```python
from build123d import *

# Parameters (mm, degrees)
SKETCH_1_W             = 10
SKETCH_1_H             = 40
SKETCH_1_R             = 1.5
EXTRUDE_1_DEPTH        = 3
SKETCH_2_W             = 1.55
SKETCH_2_H             = 40
EXTRUDE_2_DEPTH        = 3
CUT_EXTRUDE_1_DEPTH    = 3
PATTERN_LINEAR_1_COUNT = 40
PATTERN_LINEAR_1_PITCH = 1
CUT_EXTRUDE_2_DEPTH    = 10
FILLET_1_R             = 1
CUT_EXTRUDE_3_DEPTH    = 10
FILLET_2_R             = 1


with BuildPart() as part:
    # 草图1 → 凸台-拉伸1 (new body)
    with BuildSketch(Plane.XY):
        Rectangle(SKETCH_1_W, SKETCH_1_H)
        Circle(SKETCH_1_R, mode=Mode.SUBTRACT)
    extrude(amount=EXTRUDE_1_DEPTH)

    # 草图2 → 凸台-拉伸2 (add)
    with BuildSketch(Plane.XY.offset(3)):
        with Locations((-5.775, 0)):
            Rectangle(SKETCH_2_W, SKETCH_2_H)
    extrude(amount=-EXTRUDE_2_DEPTH)

    # 草图3 → 切除-拉伸1 (cut)
    with BuildSketch(Plane.XY.offset(3)):
        Polygon((-6.55, 19.8), (-6.05, 19.566846171), (-6.55, 19.333692342), align=None)
    cut_extrude_1 = extrude(amount=-CUT_EXTRUDE_1_DEPTH, mode=Mode.SUBTRACT)

    # 阵列(线性)1: 切除-拉伸1 ×40
    with Locations(*[(0, -i * PATTERN_LINEAR_1_PITCH, 0) for i in range(1, PATTERN_LINEAR_1_COUNT)]):
        add(cut_extrude_1, mode=Mode.SUBTRACT)

    # 草图5 → 切除-拉伸2 (cut)
    with BuildSketch(Plane.XY.offset(3)):
        Polygon((-0.5, 20), (-0.5, 8.485281374), (-5, 3), (-5.480467746, 6.547419937), (-7.040068743, 6.547419937), (-7.040068743, 9.445607815), (-8.18437591, 20), align=None)
    extrude(amount=-CUT_EXTRUDE_2_DEPTH, mode=Mode.SUBTRACT)

    # 圆角1
    fillet_1_edges = [part.edges().sort_by_distance(p)[0] for p in [
        (-0.5, 8.485281374, 1.5),
        (-5, 3, 1.5),
    ]]
    fillet(fillet_1_edges, radius=FILLET_1_R)

    # 草图7 → 切除-拉伸3 (cut)
    with BuildSketch(Plane(origin=(0, 0, 0), x_dir=(-1, 0, 0), z_dir=(0, 0, -1))):
        with BuildLine():
            Line((6.55, -20), (-5.418170251, -22.566873238))
            Line((-5.418170251, -22.566873238), (-10.062870934, -14.075772272))
            Line((-10.062870934, -14.075772272), (-5, -10.23011241))
            add(Edge.make_bspline(
                [(-5, -10.23011241), (-3.025837533, -19.554793567), (6.55, -20)],
                knots=[0, 0, 0, 1, 1, 1], degree=2))
        make_face()
    extrude(amount=-CUT_EXTRUDE_3_DEPTH, mode=Mode.SUBTRACT)

    # 圆角2
    fillet_2_edges = [part.edges().sort_by_distance(p)[0] for p in [
        (-0.5, 20, 1.5),
        (5, 20, 1.5),
    ]]
    fillet(fillet_2_edges, radius=FILLET_2_R)


solid = part.part
```
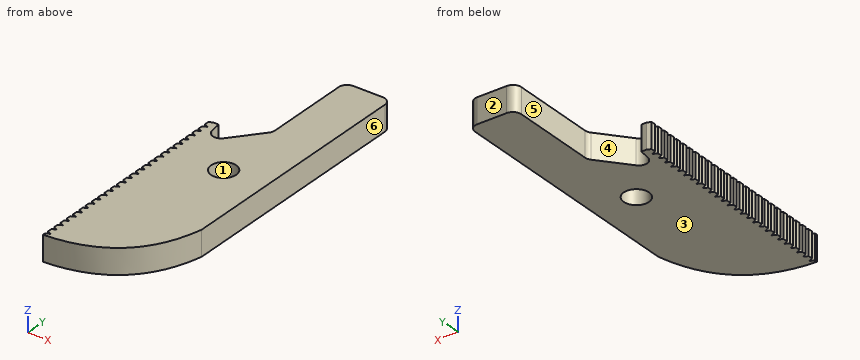
The model under review builds one solid part; all positions refer to its coordinate system, in mm. Face numbers are marked on the shaded views. A direction names the side the tool comes from. Round coordinates to 2 decimals unless told otherwise and drop trailing zeros. Loops run counter-clockwise (first coordinate to the right, second up) from the corner with the lowest first, then second, coordinate; pieces in that order, holes last. Notation, with made-up numbers: (-0.5, 54.25) - (18.5, 54.25) arc R21 cw to (18.5, 66.25) - close; hole circle Ø7 at (28, 29). An arc over 180 degrees is marked (long way). Use a Markdown table: item, result. Add a question column.
Q1. Machinability: for the marked faces 4, 5 and 6, which of the approach directions +Z, -Z, +X, -X, +Y, -Y give a long, thin tool a straight path to every point of the face, cutting with its end or side? Answer none if there is none.
Q2. Add section A-A (y = 7). State the section outline as (x, z) points, plus the area to 3 significant figures.
Q3. Insertion check: pin 1 Ø0.7 at (x, z) = (-5.5, 1.5) entering from +Y. The pin has a flat end and moves straight along its axis. Give the tip position at first contact, or say it passes through.
Q4. For probe 1 along Y at (x, z) = (0, 1.05); probe 2 along X at (y, z) = (17, 0.3); probe 3 along X at (y, z) = (4.5, 2.35), list the stretches that pass through material, from the lowest coordinate up.
Q5. The part is to be moulded in two halves that separate along Y. For the marked faces 1, 2 and 3, say which applies: pulls with the +Y half, pulls with the -Y half, needs draft (parallel to the pull), parting line crosses it, or undercut.
Worked answers:
| question | item | result |
|---|---|---|
| 1 | face 4 | +Z, -Z, +Y |
| 1 | face 5 | +Z, -Z, -X, +Y |
| 1 | face 6 | +Z, -Z, +X, +Y, -Y |
| 2 | outline | (-1.72, 0) - (5, 0) - (5, 3) - (-1.72, 3) - close |
| 2 | area | 20.2 mm² |
| 3 | pin 1 | y = 6.55 |
| 4 | probe 1 | -18.16 to -1.5, 1.5 to 19.87 |
| 4 | probe 2 | -0.5 to 5 |
| 4 | probe 3 | -6.19 to -4.73, -3.9 to 5 |
| 5 | face 1 | undercut |
| 5 | face 2 | pulls with the +Y half |
| 5 | face 3 | needs draft |
